Part model, mm, in its own coordinate system. Face numbers are marked on the shaded views. A direction names the side the tool comes from. Coordinates: 2 decimals unless noted, no trailing zeros. Order: outer loops, then holes, each group sorted by start corner. A loop starts at its lowest first (then second) coordinate and runs counter-clockwise, first axis right, second up.
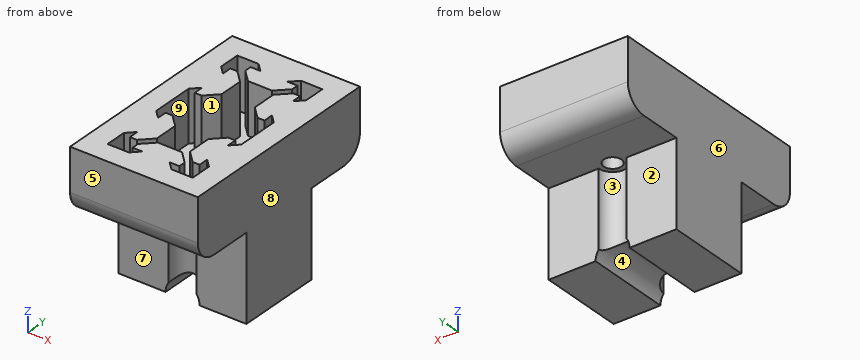
Solid Edge part; units mm, degrees
sketch "Sketch1" plane through (0, 0, 0) normal (0, -1, 0) x (1, 0, 0)
  line L0 (-15, 20) -> (-15, 0)
  line L1 (-15, 0) -> (-4, 0)
  line L2 (4, 0) -> (15, 0)
  line L3 (15, 0) -> (15, 20)
  line L4 (-15, 20) -> (15, 20)
  arc A0 (-4, 0) -> (4, 0) centre (0, 0) cw
extrude "Protrusion1" add sketch "Sketch1" against normal blind 30
sketch "Sketch2" plane through (0, 15, 20) normal (0, 0, 1) x (1, 0, 0)
  line L0 (-15, -25) -> (15, -25)
  line L1 (15, -25) -> (15, 25)
  line L2 (15, 25) -> (-15, 25)
  line L3 (-15, 25) -> (-15, -25)
extrude "ExtrudedProtrusion_2" add sketch "Sketch2" along normal blind 15
fillet "Round_1" radius 5 1 edges at (0, -10, 20)
sketch "Sketch3" plane through (15, 15, 17.5) normal (1, 0, 0) x (0, 1, 0)
  line L0 (10, -17.5) -> (10, 2.5)
  line L1 (10, 2.5) -> (15, 2.5)
  line L2 (15, 2.5) -> (15, -17.5)
  line L3 (15, -17.5) -> (10, -17.5)
  line L4 (-10, 2.5) -> (-10, -17.5)
  line L5 (-10, -17.5) -> (-15, -17.5)
  line L6 (-15, -17.5) -> (-15, 2.5)
  line L7 (-15, 2.5) -> (-10, 2.5)
extrude "Cutout1" cut sketch "Sketch3" against normal blind 30
fillet "Round_4" radius 5 1 edges at (0, 40, 20)
sketch "Sketch4" plane through (0, 15, 35) normal (0, 0, 1) x (0, 1, 0)
  line L0 (4.5007, -6.56) -> (7.16, -3.9007)
  line L1 (12.84, -3.9007) -> (7.16, -3.9007)
  line L2 (15.4993, -6.56) -> (12.84, -3.9007)
  line L3 (15.4993, -8.2) -> (15.4993, -6.56)
  line L4 (13.2, -8.2) -> (15.4993, -8.2)
  line L5 (15, -10) -> (13.2, -8.2)
  line L6 (20, -10) -> (15, -10)
  line L7 (20, -10) -> (20, -5)
  line L8 (20, -5) -> (18.2, -3.2)
  line L9 (18.2, -3.2) -> (18.2, -5.4993)
  line L10 (18.2, -5.4993) -> (16.56, -5.4993)
  line L11 (16.56, -5.4993) -> (13.9007, -2.84)
  line L12 (13.9007, 2.84) -> (13.9007, -2.84)
  line L13 (16.56, 5.4993) -> (13.9007, 2.84)
  line L14 (18.2, 5.4993) -> (16.56, 5.4993)
  line L15 (18.2, 3.2) -> (18.2, 5.4993)
  line L16 (20, 5) -> (18.2, 3.2)
  line L17 (20, 10) -> (20, 5)
  line L18 (20, 10) -> (15, 10)
  line L19 (15, 10) -> (13.2, 8.2)
  line L20 (13.2, 8.2) -> (15.4993, 8.2)
  line L21 (15.4993, 8.2) -> (15.4993, 6.56)
  line L22 (15.4993, 6.56) -> (12.84, 3.9007)
  line L23 (12.84, 3.9007) -> (7.16, 3.9007)
  line L24 (4.5007, 6.56) -> (7.16, 3.9007)
  line L25 (4.5007, 8.2) -> (4.5007, 6.56)
  line L26 (6.8, 8.2) -> (4.5007, 8.2)
  line L27 (5, 10) -> (6.8, 8.2)
  line L28 (0, 10) -> (5, 10)
  line L29 (0, 10) -> (-5, 10)
  line L30 (-5, 10) -> (-6.8, 8.2)
  line L31 (-6.8, 8.2) -> (-4.5007, 8.2)
  line L32 (-4.5007, 8.2) -> (-4.5007, 6.56)
  line L33 (-4.5007, 6.56) -> (-7.16, 3.9007)
  line L34 (-12.84, 3.9007) -> (-7.16, 3.9007)
  line L35 (-15.4993, 6.56) -> (-12.84, 3.9007)
  line L36 (-15.4993, 8.2) -> (-15.4993, 6.56)
  line L37 (-13.2, 8.2) -> (-15.4993, 8.2)
  line L38 (-15, 10) -> (-13.2, 8.2)
  line L39 (-20, 10) -> (-15, 10)
  line L40 (-20, 10) -> (-20, 5)
  line L41 (-20, 5) -> (-18.2, 3.2)
  line L42 (-18.2, 3.2) -> (-18.2, 5.4993)
  line L43 (-18.2, 5.4993) -> (-16.56, 5.4993)
  line L44 (-16.56, 5.4993) -> (-13.9007, 2.84)
  line L45 (-13.9007, 2.84) -> (-13.9007, -2.84)
  line L46 (-16.56, -5.4993) -> (-13.9007, -2.84)
  line L47 (-18.2, -5.4993) -> (-16.56, -5.4993)
  line L48 (-18.2, -3.2) -> (-18.2, -5.4993)
  line L49 (-20, -5) -> (-18.2, -3.2)
  line L50 (-20, -10) -> (-20, -5)
  line L51 (-20, -10) -> (-15, -10)
  line L52 (-15, -10) -> (-13.2, -8.2)
  line L53 (-13.2, -8.2) -> (-15.4993, -8.2)
  line L54 (-15.4993, -8.2) -> (-15.4993, -6.56)
  line L55 (-15.4993, -6.56) -> (-12.84, -3.9007)
  line L56 (-12.84, -3.9007) -> (-7.16, -3.9007)
  line L57 (-4.5007, -6.56) -> (-7.16, -3.9007)
  line L58 (-4.5007, -8.2) -> (-4.5007, -6.56)
  line L59 (-6.8, -8.2) -> (-4.5007, -8.2)
  line L60 (-5, -10) -> (-6.8, -8.2)
  line L61 (0, -10) -> (-5, -10)
  line L62 (0, -10) -> (5, -10)
  line L63 (5, -10) -> (6.8, -8.2)
  line L64 (6.8, -8.2) -> (4.5007, -8.2)
  line L65 (4.5007, -8.2) -> (4.5007, -6.56)
extrude "ExtrudedCutout_7" cut sketch "Sketch4" against normal blind 12
sketch "Sketch5" plane through (0, 15, 35) normal (0, 0, 1) x (0, 1, 0)
  circle A0 centre (-10, 0) radius 2.1
  circle A1 centre (10, 0) radius 2.1
extrude "ExtrudedCutout_8" cut sketch "Sketch5" against normal blind 50
sketch "Sketch6" plane through (0, 30, 20) normal (0, 0, -1) x (0, 1, 0)
  circle A0 centre (-5, 0) radius 3.25
  circle A1 centre (-25, 0) radius 3.25
extrude "ExtrudedCutout_9" cut sketch "Sketch6" along normal blind 30
extrude "ExtrudedCutout_1" [suppressed]
extrude "ExtrudedCutout_2" [suppressed]
extrude "ExtrudedCutout_4" [suppressed]
extrude "ExtrudedCutout_5" [suppressed]
fillet "Round_2" [suppressed]
(1) Slice it at C-C, the plane x = 13.25. Give the cut face in (y, z), then the cut area to 3 significant figures.
(2) Drop flat-ended pins along their axis: pin 1 (12 mm diameter, centred on x = -7, z = 4, fed in from +Y); pin 2 (3.5 mm diameter, centred on x = -10.5, z = 15, fed in from -Y); pin 3 (6 mm diameter, centred on x = 2, y = 29, fed in from -Z). Give the stop position or say it passes through.
(3) Pull direction X, two halves, no side cores. Call the marked faces 6, 7, 8 and 9: +X half, -X half, draft (parallel to the pull), parting line (faces both ways), or undercut.
(4) Tool access for the marked faces 1, 2, 3, 4 and 5: list every direction of +Z, -Z, +X, -X, +Y, -Y with a clear straight run to the whole face (end or side of a thin tool).
(5) Slice it at A-A, the plane x = 0. Give the cut face in (y, z), then the cut area to 3 significant figures.
(6) Slice it at B-B, the plane y = 12.5. Give the cut face in (x, z).
(7) Slice it at D-D, the plane z = 8. Give the cut face in (x, y).
(8) Probe line 1 (Y direction, x = 8, z = 27); line 2 (X direction, y = 5, z = 21.4); line 3 (Y direction, x = -4.25, z = 28). List the from-to ranges inside material, lowest first.
Here are the results:
1. outline: (-10, 25) arc R5 ccw to (-5, 20) - (5, 20) - (5, 0) - (25, 0) - (25, 20) - (35, 20) arc R5 ccw to (40, 25) - (40, 35) - (-10, 35) - close
1. area: 1,140 mm2
2. pin 1: stops at y = 25
2. pin 2: stops at y = 5
2. pin 3: stops at z = 20
3. face 6: -X half
3. face 7: draft
3. face 8: +X half
3. face 9: undercut
4. face 1: +Z
4. face 2: -Z, +X, -X, +Y
4. face 3: -Z, +Y
4. face 4: -Z, +Y, -Y
4. face 5: +Z, -Z, +X, -X, -Y
5. outline: (-10, 25) arc R5 ccw to (-5, 20) - (2.9, 20) - (2.9, 23) - (1.1, 23) - (1.1, 35) - (-10, 35) - close; (7.1, 20) - (8.25, 20) - (8.25, 4) - (21.75, 4) - (21.75, 20) - (22.9, 20) - (22.9, 23) - (7.1, 23) - close; (27.1, 20) - (35, 20) arc R5 ccw to (40, 25) - (40, 35) - (28.9, 35) - (28.9, 23) - (27.1, 23) - close
5. area: 596 mm2
6. outline: (-15, 0) - (-4, 0) arc R4 cw to (4, 0) - (15, 0) - (15, 35) - (10, 35) - (10, 23) - (-10, 23) - (-10, 35) - (-15, 35) - close
7. outline: (-15, 5) - (-3.25, 5) arc R3.25 cw to (3.25, 5) - (15, 5) - (15, 25) - (3.25, 25) arc R3.25 cw to (-3.25, 25) - (-15, 25) - close
8. line 1: y = -10 to -5, -0.5 to 10.5, 19.5 to 30.5, 35 to 40
8. line 2: x = -15 to -2.1, 2.1 to 15
8. line 3: y = -10 to -4.25, -3.2 to -0.31, 1.81 to 8.19, 21.81 to 28.19, 30.31 to 33.2, 34.25 to 40
